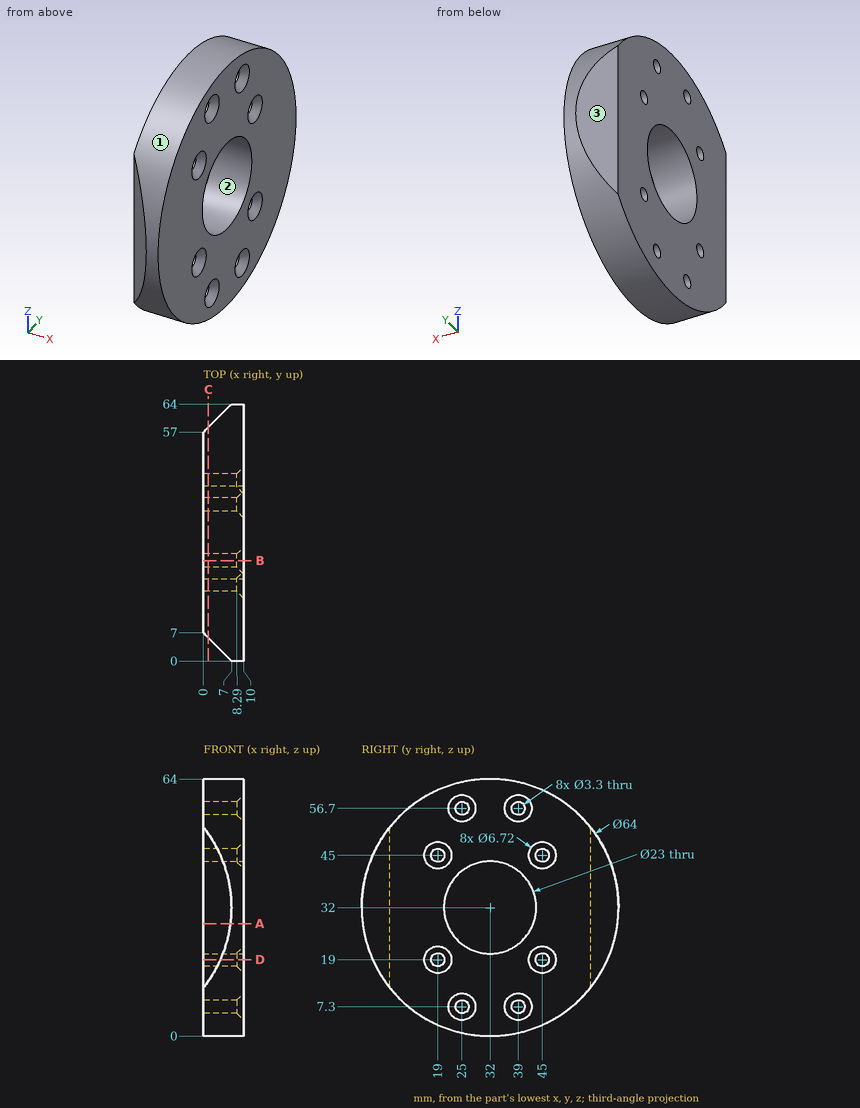
For this review, use the dimensioned drawing (mm, ordinates from the lowest corner) and the shaded views. Give positions to 0.01 mm unless a question says otherwise; leave off trailing zeros. Loops run counter-clockwise (first coordinate to the right, second up) from the corner with the lowest first, then second, coordinate; pieces in that order, holes last.
Item 1: For line 1 along Y through (x, z) = (2, 56.7); line 2 along Z through (x, y) = (4.5, 45); line 3 along Y through (x, z) = (4, 19), list the stretches that pass through material, from the lowest coordinate up.
Item 2: Take a section at C-C, the plane x = 1.25. Give the number of separate pieces and of enclosed holes in the cut face, and give its area (3 significant figures).
Item 3: Take a section at A-A, the plane z = 28. State the section outline as (x, y) points, and give its area (3 significant figures).
Item 4: Draft analysis for pull direction Z (two halves, no side actions). For the marked faces 1, 2 and 3, state which applies: +Z half, -Z half, draft (parallel to the pull), parting line (faces both ways), or undercut.
Item 5: Insertion check: pin 1 (3 mm diameter, centred on x = 8.5, z = 12.5, fed in from +Y); pin 2 (4.5 mm diameter, centred on y = 19, z = 45, fed in from +X); pin 3 (1 mm diameter, centred on x = 5.5, y = 52, fed in from -Z). Each pin has a flat end and moves straight along its axis. Give the tip position at first contact, or say it passes through.
Item 6: Take a section at B-B, the plane y = 25. State the section outline as (x, z) points, and give its area (3 significant figures).
Item 7: Take a section at D-D, the plane z = 19. State the section outline as (x, y) points.
Calculated:
1. line 1: y = 11.66 to 23.35, 26.65 to 37.35, 40.65 to 52.34
1. line 2: z = 2.76 to 17.35, 20.65 to 43.35, 46.65 to 61.24
1. line 3: y = 3 to 17.35, 20.65 to 43.35, 46.65 to 61
2. separate pieces: 1
2. enclosed holes: 9
2. area: 2,450 mm2
3. outline: (0, 7) - (6.75, 0.25) - (10, 0.25) - (10, 21.22) - (0, 21.22) - close; (0, 42.78) - (10, 42.78) - (10, 63.75) - (6.75, 63.75) - (0, 57) - close
3. area: 374 mm2
4. face 1: parting line
4. face 2: undercut
4. face 3: draft
5. pin 1: stops at y = 58.46
5. pin 2: stops at x = 8.89
5. pin 3: stops at z = 6.63
6. outline: (0, 0.78) - (10, 0.78) - (10, 3.94) - (8.29, 5.65) - (0, 5.65) - close; (0, 8.95) - (8.29, 8.95) - (10, 10.66) - (10, 22.88) - (0, 22.88) - close; (0, 41.12) - (10, 41.12) - (10, 53.34) - (8.29, 55.05) - (0, 55.05) - close; (0, 58.35) - (8.29, 58.35) - (10, 60.06) - (10, 63.22) - (0, 63.22) - close
6. area: 370 mm2
7. outline: (0, 7) - (4.24, 2.76) - (10, 2.76) - (10, 15.64) - (8.29, 17.35) - (0, 17.35) - close; (0, 20.65) - (8.29, 20.65) - (10, 22.36) - (10, 41.64) - (8.29, 43.35) - (0, 43.35) - close; (0, 46.65) - (8.29, 46.65) - (10, 48.36) - (10, 61.24) - (4.24, 61.24) - (0, 57) - close
